Geometry: see drawing. Coordinates: mm, zero at the bounding-box minimum. Give positions to 0.01 mm unless a question says otherwise; leave off trailing zeros. Write each loop counter-clockwise with the first axis right and the second up, starting at its lowest first coordinate (ties: lowest second). Pieces come first, ordered by that corner, then holes. Notation, with made-up numbers: M 89,-23 L 137,-23 A16 ccw 137,-10 Z; hole C 59.5,-21.75 d5. An arc over 180 degrees is marked long. Use a Markdown table: item, result. Add a question column.
(1) Cut plane A-A (y = 14.75). Output: boundary loops of the cut face in (x, z) (1 decimal), plus the area to 3 significant figures.
(2) Pin query (flat end, axial travel): pin 1 Ø1.5 at (y, z) = (13, 104.5) entering from -X (1 decimal); pin 2 Ø10 at (y, z) = (2, 74) entering from -X (1 decimal); pin 3 Ø1 at (y, z) = (6, 186.5) entering from +X; pin 4 Ø12 at (x, z) = (536.78, 212.5) entering from +Y. Return the tip coordinate at first contact, or that it passes through.
(3) Material intervals for L1, parallel to Z at x = 393, y = 5.25; L2, parallel to Z at x = 161, y = 14.5 (1 decimal); L3, parallel to X at y = 15, z = 18, sorted ascending.
(4) Cut plane B-B (z = 212.5). Output: boundary loops of the cut face in (x, y), plus the area to 3 significant figures.
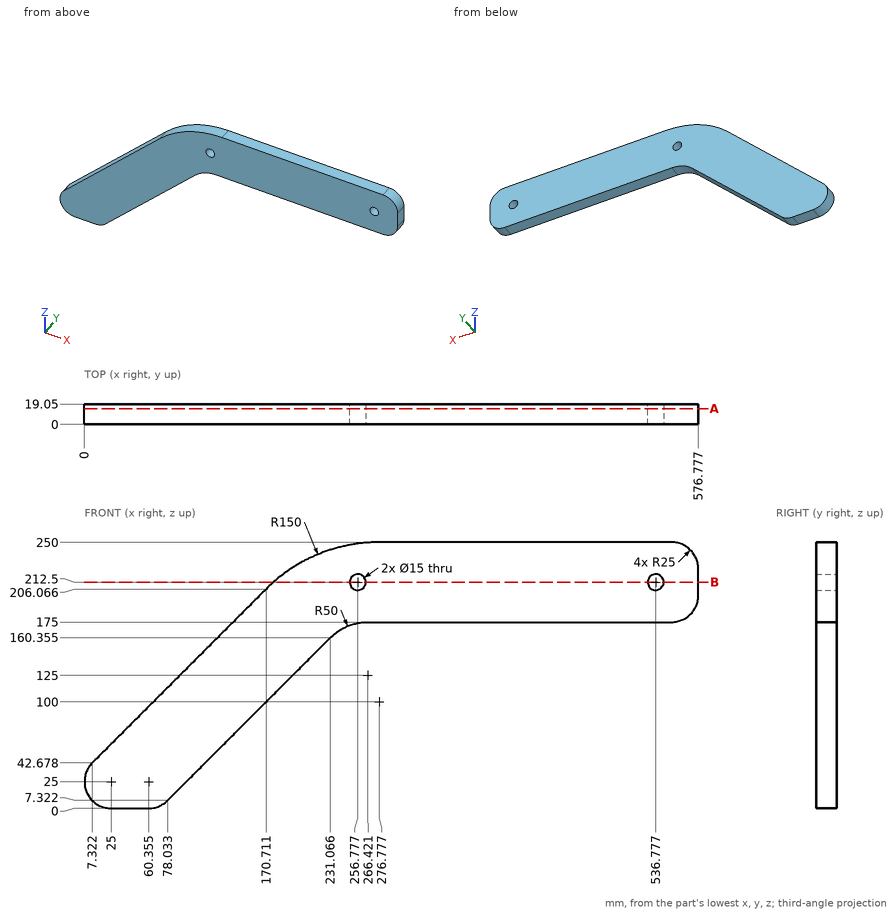
Answer list:
| question | item | result |
|---|---|---|
| 1 | outline | M 7.3,42.7 A25 ccw 25,0 L 60.4,0 A25 ccw 78,7.3 L 231.1,160.4 A50 cw 266.4,175 L 551.8,175 A25 ccw 576.8,200 L 576.8,225 A25 ccw 551.8,250 L 276.8,250 A150 ccw 170.7,206.1 Z; hole C 256.8,212.5 d15; hole C 536.8,212.5 d15 |
| 1 | area | 46,700 mm² |
| 2 | pin 1 | x = 68.4 |
| 2 | pin 2 | x = 33.6 |
| 2 | pin 3 | x = 573.13 |
| 2 | pin 4 | through |
| 3 | L1 | 175 to 250 |
| 3 | L2 | 90.3 to 196.4 |
| 3 | L3 | 1 to 88.71 |
| 4 | outline | M 177.56,0 L 249.28,0 L 249.28,19.05 L 177.56,19.05 Z; M 264.28,0 L 529.28,0 L 529.28,19.05 L 264.28,19.05 Z; M 544.28,0 L 576.78,0 L 576.78,19.05 L 544.28,19.05 Z |
| 4 | area | 7,030 mm² |
